from build123d import *

# Parameters (mm, degrees)
BASE_DEPTH             = 146
HINGE_CUT_DEPTH        = 43
HINGE_START            = -103
HINGE_CUT_2_DEPTH      = 43
HINGE_START_2          = -62
SKETCH3_R              = 0.75
HINGE_EXTRUSIONS_DEPTH = 64
FILLET5_R              = 0.5
FILLET6_R              = 0.5
SYRINGE_START          = -92
SYRINGE_HOLDER_DEPTH   = 2
LPATTERN4_COUNT        = 2
LPATTERN4_PITCH        = 40
FILLET7_R              = 1
FILLET8_R              = 0.5
SNAP_START             = -12.431858348
SNAP_GROOVE1_DEPTH     = 2
SNAP_START_2           = -13.062831461
SNAP_GROOVE1_2_DEPTH   = 0.630973113
LPATTERN5_COUNT        = 2
LPATTERN5_PITCH        = 81
SKETCH6_W              = 6.31577628
SKETCH6_H              = 38
VISIBILITY_DEPTH       = 2
SKETCH7_W              = 6.177782062
SKETCH7_H              = 12
CUT_EXTRUDE4_DEPTH     = 2


# Read off the part's stored shape, not the designer's step: Snap Groove1
with BuildPart() as part:
    # Sketch1 → Base (new body)
    with BuildSketch(Plane.XY):
        with BuildLine():
            Line((0, 0), (80, 0))
            ThreePointArc((80, 0), (89.545941546, 3.954058454), (93.5, 13.5))
            ThreePointArc((93.5, 13.5), (92.5, 13.70219929), (91.5, 13.5))
            ThreePointArc((91.5, 13.5), (88.131727984, 5.368272016), (80, 2))
            Line((80, 2), (0, 2))
            ThreePointArc((0, 2), (-8.131727984, 5.368272016), (-11.5, 13.5))
            Line((-11.5, 13.5), (-13.5, 13.5))
            ThreePointArc((-13.5, 13.5), (-9.545941546, 3.954058454), (0, 0))
        make_face()
    extrude(amount=-BASE_DEPTH)

    # Sketch2 → Hinge cut (cut)
    with BuildSketch(Plane.XY):
        with BuildLine():
            ThreePointArc((93.5, 13.5), (93.179996096, 10.578065212), (92.235155125, 7.794653467))
            ThreePointArc((92.235155125, 7.794653467), (91.53133512, 8.651508178), (90.422539551, 8.63988999))
            ThreePointArc((90.422539551, 8.63988999), (91.227404082, 11.01094444), (91.5, 13.5))
            ThreePointArc((91.5, 13.5), (92.5, 13.914213562), (93.5, 13.5))
        make_face()
    extrude(amount=-HINGE_CUT_DEPTH, mode=Mode.SUBTRACT)

    # Sketch2<2> → Hinge cut 2 (cut)
    with BuildSketch(Plane.XY.offset(HINGE_START)):
        with BuildLine():
            ThreePointArc((93.5, 13.5), (93.179996096, 10.578065212), (92.235155125, 7.794653467))
            ThreePointArc((92.235155125, 7.794653467), (91.53133512, 8.651508178), (90.422539551, 8.63988999))
            ThreePointArc((90.422539551, 8.63988999), (91.227404082, 11.01094444), (91.5, 13.5))
            ThreePointArc((91.5, 13.5), (92.5, 13.914213562), (93.5, 13.5))
        make_face()
    extrude(amount=-HINGE_CUT_2_DEPTH, mode=Mode.SUBTRACT)

    # Sketch3 → hinge extrusions (add)
    with BuildSketch(Plane.XY.offset(-43).offset(HINGE_START_2)):
        with Locations(Location((92.3, 12, 0), (0, 0, 180))):
            Circle(SKETCH3_R)
    extrude(amount=HINGE_EXTRUSIONS_DEPTH)

    # Fillet5
    fillet5_edges = [part.edges().sort_by_distance(p)[0] for p in [
        (93.05, 12, -105),
    ]]
    fillet(fillet5_edges, radius=FILLET5_R)

    # Fillet6
    fillet6_edges = [part.edges().sort_by_distance(p)[0] for p in [
        (93.05, 12, -41),
    ]]
    fillet(fillet6_edges, radius=FILLET6_R)

    # Sketch5 → Syringe holder (add)
    with BuildSketch(Plane(origin=(0, 0, -146), x_dir=(-1, 0, 0), z_dir=(0, 0, -1)).offset(SYRINGE_START)):
        with BuildLine():
            Line((0, 2), (-1.5, 2))
            Line((-1.5, 2), (-1.5, 9))
            ThreePointArc((-1.5, 9), (0.0084764, 8.790290315), (1.5, 9.098245749))
            Line((1.5, 9.098245749), (1.5, 2.098245749))
            ThreePointArc((1.5, 2.098245749), (0.751606983, 2.024587722), (0, 2))
        make_face()
    syringe_holder = extrude(amount=SYRINGE_HOLDER_DEPTH)

    # LPattern4: Syringe holder ×2
    with Locations(*[(0, 0, i * LPATTERN4_PITCH) for i in range(1, LPATTERN4_COUNT)]):
        add(syringe_holder)

    # Fillet7
    fillet7_edges = [part.edges().sort_by_distance(p)[0] for p in [
        (92.235155125, 7.794653467, -21.5),
        (90.422539551, 8.63988999, -21.5),
        (92.235155125, 7.794653467, -124.5),
        (90.422539551, 8.63988999, -124.5),
    ]]
    fillet(fillet7_edges, radius=FILLET7_R - 0.0001)  # a hair under: the kernel refuses the full size

    # Fillet8
    fillet8_edges = [part.edges().sort_by_distance(p)[0] for p in [
        (93.5, 13.5, -73),
        (91.5, 13.5, -73),
    ]]
    fillet(fillet8_edges, radius=FILLET8_R)

    # Snap Groove1 outline → Snap Groove1 (cut)
    with BuildSketch(Plane(origin=(0, 0, 0), x_dir=(0.0006419218138647702, 0.9999997939681713, 0), z_dir=(0.9999997939681713, -0.0006419218138647702, 0)).offset(SNAP_START)):
        Polygon((8.059246911, -107.890634842), (12.059246911, -108.100265959), (12.059246911, -105.681003725), (8.059246911, -105.890634842), align=None)
    snap_groove1 = extrude(amount=SNAP_GROOVE1_DEPTH, mode=Mode.SUBTRACT)

    # Snap Groove1 2 outline → Snap Groove1 2 (cut)
    with BuildSketch(Plane(origin=(0, 0, 0), x_dir=(0.0006419218138647702, 0.9999997939681713, 0), z_dir=(0.9999997939681713, -0.0006419218138647702, 0)).offset(SNAP_START_2)):
        Polygon((8.059246911, -107.890634842), (10.059246911, -107.9954504), (10.059246911, -105.785819283), (8.059246911, -105.890634842), align=None)
    snap_groove1_2 = extrude(amount=SNAP_GROOVE1_2_DEPTH, mode=Mode.SUBTRACT)

    # LPattern5: Snap Groove1, Snap Groove1 2 ×2
    with Locations(*[(0, 0, i * LPATTERN5_PITCH) for i in range(1, LPATTERN5_COUNT)]):
        add(snap_groove1, mode=Mode.SUBTRACT)
        add(snap_groove1_2, mode=Mode.SUBTRACT)

    # Sketch6 → Visibility (cut)
    with BuildSketch(Plane(origin=(0, 2, 0), x_dir=(1, 0, 0), z_dir=(0, 1, 0))):
        with Locations((3.15788814, 35)):
            Rectangle(SKETCH6_W, SKETCH6_H)
    extrude(amount=-VISIBILITY_DEPTH, mode=Mode.SUBTRACT)

    # Sketch7 → Cut-Extrude4 (cut)
    with BuildSketch(Plane(origin=(0, 2, 0), x_dir=(1, 0, 0), z_dir=(0, 1, 0))):
        with Locations((3.088891031, 8)):
            Rectangle(SKETCH7_W, SKETCH7_H)
    extrude(amount=-CUT_EXTRUDE4_DEPTH, mode=Mode.SUBTRACT)


solid = part.part
The listing builds one solid part. Answer for the finished solid, in the listing's coordinates (mm). A direction names the side the tool comes from. Round coordinates to 2 decimals unless told otherwise and drop trailing zeros. Order: outer loops, then holes, each group sorted by start corner. A loop starts at its lowest first (then second) coordinate and runs counter-clockwise, first axis right, second up. Notation, with made-up numbers: (26.5, -4) -> (83.5, -4) arc R20 ccw to (83.5, 19) -> close; hole circle Ø1 at (-5, -32.75). An arc over 180 degrees is marked (long way). Put each result on its own line as item: value.
Q1. Consider line 1 along Y through (x, z) = (33.5, -90); line 2 along X through (y, z) = (12, -71); line 3 along X through (y, z) = (8.5, -32). Determine where each line is inside the solid, lowest interval first.
Results list:
line 1: 0 to 2
line 2: -13.42 to -11.4, 91.4 to 93.42
line 3: -12.54 to -10.36, 90.44 to 91.76
Q2. Determine the mould class of faces 1 (the flat face through (35.1, 1.8, 0)), 2 (the flat face through (39, 0, -72)), 3 (the flat face through (92, 11, -103)), 4 (the flat face through (92, 11, -43)) for opening direction Y: pulls with the +Y half, pulls with the -Y half, needs draft (parallel to the pull), parting line crosses it, or undercut.
Results list:
face 1: needs draft
face 2: pulls with the -Y half
face 3: undercut
face 4: undercut
Q3. Section A-A, the plane y = 4.75 is taken. Write down the section's boundary in (x, z), and give its area (3 significant figures).
Results list:
outline: (-10.28, -146) -> (-7.46, -146) -> (-7.46, 0) -> (-10.28, 0) -> close; (-1.5, -56) -> (1.5, -56) -> (1.5, -54) -> (-1.5, -54) -> close; (-1.5, -16) -> (1.5, -16) -> (1.5, -14) -> (-1.5, -14) -> close; (87.46, -146) -> (90.28, -146) -> (90.28, 0) -> (87.46, 0) -> close
area: 835 mm^2
Q4. Which of the six approach directions +Z, -Z, +X, -X, +Y, -Y give full straight-line access (tool end or side, diameter ignored) to faces 5 (the flat face through (35.1, 1.8, -146)), 6 (the flat face through (1, 4, -16)), 7 (the cylindrical face through (86.588, 4.074, -71.978)), 8 (the cylindrical face through (-9.65, 4.06, -71.98)), 9 (the flat face through (0, 6, -56))?
Results list:
face 5: -Z, +X, -X, +Y, -Y
face 6: +Y
face 7: +Z, -Z, +Y
face 8: +Z, -Z, -X, -Y
face 9: -Z, +Y
Q5. Each of these flat-tipped pins is pushed along its axis until it touches: P1, Ø1.6, axis at x = 92, y = 11.5, coming from the -Z side; P2, Ø1, axis at x = 26.5, y = 1.5, coming from the +Z side; P3, Ø1.5, axis at x = -1.5, y = 9.5, coming from the +Z side; P4, Ø1, axis at y = 0.5, z = -9.5, coming from the -X side. Where does it stop, or does it pass through?
Results list:
P1: z = -105
P2: z = 0
P3: z = -14
P4: x = -5.1
